```python
from build123d import *

# Parameters (mm, degrees)
F0_R     = 3.175
F0_R_2   = 2.8227407603
F0_R_3   = 2.8948343133
F1_DEPTH = 25.4


with BuildPart() as f1:
    # F0 (on Front) → F1 (new body)
    with BuildSketch(Plane.XZ):
        with BuildLine():
            ThreePointArc((-9.525, 114.3), (0, 104.775), (9.525, 114.3))
            ThreePointArc((9.525, 114.3), (0, 123.825), (-9.525, 114.3))
        make_face()
        with Locations((0, 114.3)):
            Circle(F0_R, mode=Mode.SUBTRACT)
        with BuildLine():
            Line((15.487804878, 60.6347560976), (9.525, 114.3))
            ThreePointArc((9.525, 114.3), (0, 104.775), (-9.525, 114.3))
            Line((-9.525, 114.3), (-15.487804878, 60.6347560976))
            ThreePointArc((-15.487804878, 60.6347560976), (0, 73.025), (15.487804878, 60.6347560976))
        make_face()
        with Locations((-4.7098048963, 93.5786440969)):
            Circle(F0_R_2, mode=Mode.SUBTRACT)
        with BuildLine():
            Line((15.875, 57.15), (15.487804878, 60.6347560976))
            ThreePointArc((15.487804878, 60.6347560976), (0, 73.025), (-15.487804878, 60.6347560976))
            Line((-15.487804878, 60.6347560976), (-15.875, 57.15))
            Line((-15.875, 57.15), (-15.487804878, 53.6652439024))
            ThreePointArc((-15.487804878, 53.6652439024), (0, 41.275), (15.487804878, 53.6652439024))
            Line((15.487804878, 53.6652439024), (15.875, 57.15))
        make_face()
        with Locations((0, 57.15)):
            Circle(F0_R, mode=Mode.SUBTRACT)
        with BuildLine():
            ThreePointArc((15.875, 57.15), (15.7779042879, 58.9031004764), (15.487804878, 60.6347560976))
            Line((15.487804878, 60.6347560976), (15.875, 57.15))
        make_face()
        with BuildLine():
            Line((-15.875, 57.15), (-15.487804878, 60.6347560976))
            ThreePointArc((-15.487804878, 60.6347560976), (-15.7779042879, 58.9031004764), (-15.875, 57.15))
        make_face()
        with BuildLine():
            ThreePointArc((15.487804878, 53.6652439024), (15.7779042879, 55.3968995236), (15.875, 57.15))
            Line((15.875, 57.15), (15.487804878, 53.6652439024))
        make_face()
        with BuildLine():
            Line((-15.487804878, 53.6652439024), (-15.875, 57.15))
            ThreePointArc((-15.875, 57.15), (-15.7779042879, 55.3968995236), (-15.487804878, 53.6652439024))
        make_face()
        with BuildLine():
            Line((11.2837349209, 15.8286142885), (15.487804878, 53.6652439024))
            ThreePointArc((15.487804878, 53.6652439024), (0, 41.275), (-15.487804878, 53.6652439024))
            Line((-15.487804878, 53.6652439024), (-9.525, 0))
            ThreePointArc((-9.525, 0), (0, 9.525), (9.525, 0))
            ThreePointArc((9.525, 0), (7.2595482465, -6.1664077271), (1.5408353267, -9.3995452813))
            Line((1.5408353267, -9.3995452813), (44.45, -5.9058837015))
            ThreePointArc((44.45, -5.9058837015), (38.545468302, 0.1263634545), (44.7026690535, 5.9004763066))
            Line((44.7026690535, 5.9004763066), (18.8451791707, 7.0077407296))
            ThreePointArc((18.8451791707, 7.0077407296), (13.1493027106, 9.7764656492), (11.2837349209, 15.8286142885))
        make_face()
        with BuildLine():
            Line((0, 0), (-9.525, 0))
            ThreePointArc((-9.525, 0), (-6.7351920908, -6.7351920908), (0, -9.525))
            Line((0, -9.525), (0, 0))
        make_face()
        with BuildLine():
            ThreePointArc((9.525, 0), (0, 9.525), (-9.525, 0))
            Line((-9.525, 0), (0, 0))
            Line((0, 0), (0, -9.525))
            Line((0, -9.525), (1.5408353267, -9.3995452813))
            ThreePointArc((1.5408353267, -9.3995452813), (7.2595482465, -6.1664077271), (9.525, 0))
        make_face()
        with BuildLine():
            Line((1.5408353267, -9.3995452813), (0, -9.525))
            ThreePointArc((0, -9.525), (0.7729670741, -9.4935845128), (1.5408353267, -9.3995452813))
        make_face()
        with BuildLine():
            ThreePointArc((50.3558837015, 0), (48.7144868589, 4.0857819478), (44.7026690535, 5.9004763066))
            ThreePointArc((44.7026690535, 5.9004763066), (38.545468302, 0.1263634545), (44.45, -5.9058837015))
            ThreePointArc((44.45, -5.9058837015), (48.6260904142, -4.1760904142), (50.3558837015, 0))
        make_face()
        with Locations((44.45, 0)):
            Circle(F0_R_3, mode=Mode.SUBTRACT)
    extrude(amount=F1_DEPTH)


solid = f1.part
```
Verification items for the finished model (mm, model axes). A direction names the side the tool comes from. Coordinates: 2 decimals unless noted, no trailing zeros. Order: outer loops, then holes, each group sorted by start corner. A loop starts at its lowest first (then second) coordinate and runs counter-clockwise, first axis right, second up. Notation, with made-up numbers: (-12, -7) - (2, -7) arc R25 cw to (2, 11) - close; hole circle Ø10 at (35.5, 24.5). An arc over 180 degrees is marked (long way). Return JSON: item names as keys, results as strings.
(1) Thickness scan on line 1 along Z through (x, y) = (0, -19.5) (3 decimals); line 2 along X through (y, z) = (-14.5, 57.5); line 3 along X through (y, z) = (-23.75, 117). Record the ranges inside material, lowest first.
Filled sheet:
{"line 1": "z = -9.525 to 53.975, 60.325 to 111.125, 117.475 to 123.825", "line 2": "x = -15.87 to -3.16, 3.16 to 15.87", "line 3": "x = -9.13 to -1.67, 1.67 to 9.13"}
(2) Access from +Z, -Z, +X, -X, +Y, -Y to the whole of each face (thin tool, end or side, straight path). Record for faces 1 (the cylindrical face through (41.56, -12.52, 0.13)), 2 (the flat face through (13.356, -12.522, 34.482)).
Filled sheet:
{"face 1": "+Y, -Y", "face 2": "+X, +Y, -Y"}
(3) Section check B-B, the plane z = 99. Record the cut outline in (x, y) (3 decimals).
Filled sheet:
{"outline": "(-11.225, -25.4) - (11.225, -25.4) - (11.225, 0) - (-11.225, 0) - close"}
(4) Go/stop test with flat-tipped pins: pin 1 (2 mm diameter, centred on x = 9, y = -17, fed in from -Z); pin 2 (8 mm diameter, centred on y = -21.5, z = 20, fed in from +X); pin 3 (1.5 mm diameter, centred on x = -4, y = -11.5, fed in from -Z). Record where each tip stops, or that it passes through.
Filled sheet:
{"pin 1": "stops at z = -8.87", "pin 2": "stops at x = 12.19", "pin 3": "stops at z = -8.95"}
(5) Section check C-C, the plane x = 33. Record the cut outline in (y, z).
Filled sheet:
{"outline": "(-25.4, -6.84) - (0, -6.84) - (0, 6.4) - (-25.4, 6.4) - close"}
(6) Section check A-A, the plane y = -9.5. Record the cut outline in (x, z) (3 decimals), and give its area (3 significant figures).
Filled sheet:
{"outline": "(-15.488, 53.665) - (-9.525, 0) arc R9.525 ccw to (1.541, -9.4) - (44.45, -5.906) arc R5.906 ccw to (44.703, 5.9) - (18.845, 7.008) arc R7.95 cw to (11.284, 15.829) - (15.488, 53.665) arc R15.875 ccw to (15.488, 60.635) - (9.525, 114.3) arc R9.525 ccw to (-9.525, 114.3) - (-15.488, 60.635) arc R15.875 ccw to start; hole circle Ø5.645 at (-4.71, 93.579); hole circle Ø6.35 at (0, 57.15); hole circle Ø6.35 at (0, 114.3); hole circle Ø5.79 at (44.45, 0)", "area": "3,650 mm^2"}
